from build123d import *

# Parameters (mm, degrees)
SKETCH2_R           = 15
SKETCH2_R_2         = 10
SKETCH5_R           = 5
CUT_EXTRUDE2_DEPTH  = 158.5
SKETCH6_R           = 30
CUT_EXTRUDE3_DEPTH  = 90.8
SKETCH9_R           = 10
BOSS_EXTRUDE2_DEPTH = 211.8
SKETCH10_R          = 4.5
BOSS_EXTRUDE3_DEPTH = 10


with BuildPart() as part:
    # Sweep2: sweep along a path in Sketch1
    with BuildLine(Plane(origin=(0, 0, 0), x_dir=(0, 0, -1), z_dir=(1, 0, 0))) as sweep2_path:
        Line((0, 0), (304.8, 0))
        ThreePointArc((304.8, 0), (361.368542495, 23.431457505), (384.8, 80))
        Line((384.8, 80), (384.8, 1748.2))
        ThreePointArc((384.8, 1748.2), (361.368542495, 1804.768542495), (304.8, 1828.2))
        Line((304.8, 1828.2), (0, 1828.2))
    # Sketch2 → Sweep2 (sweep)
    with BuildSketch(Plane.XY):
        with Locations((0, 1828.2)):
            Circle(SKETCH2_R)
        with Locations((0, 1828.2)):
            Circle(SKETCH2_R_2, mode=Mode.SUBTRACT)
    sweep(path=sweep2_path.line)

    # Sketch5 → Cut-Extrude2 (cut, symmetric)
    with BuildSketch(Plane(origin=(0, 0, 0), x_dir=(1, 0, 0), z_dir=(0, 1, 0))):
        with Locations(Location((0, 30, 0), (0, 0, 270))):
            Circle(SKETCH5_R)
        with Locations(Location((0, 230, 0), (0, 0, 270))):
            Circle(SKETCH5_R)
    extrude(amount=CUT_EXTRUDE2_DEPTH, both=True, mode=Mode.SUBTRACT)

    # Sketch6 → Cut-Extrude3 (cut)
    with BuildSketch(Plane.XY):
        with Locations((0, 1828.2)):
            Circle(SKETCH6_R)
    extrude(amount=-CUT_EXTRUDE3_DEPTH, mode=Mode.SUBTRACT)

    # Sketch9 → Boss-Extrude2 (add)
    with BuildSketch(Plane.XY.offset(-90.8)):
        with Locations((0, 1828.2)):
            Circle(SKETCH9_R)
    extrude(amount=-BOSS_EXTRUDE2_DEPTH)

    # Sketch10 → Boss-Extrude3 (add)
    with BuildSketch(Plane.XY.offset(-90.8)):
        with Locations((0, 1828.2)):
            Circle(SKETCH10_R)
    extrude(amount=BOSS_EXTRUDE3_DEPTH)


solid = part.part
Could you check a few things on this model? Use its own coordinates, in mm. Coordinates: 2 decimals unless noted, no trailing zeros. Order: outer loops, then holes, each group sorted by start corner. A loop starts at its lowest first (then second) coordinate and runs counter-clockwise, first axis right, second up.
Q1. Will these pins go through, and if not, where does the flat tip stop? pin 1 (12 mm diameter, centred on x = -12, z = -170, fed in from +Y); pin 2 (1.5 mm diameter, centred on x = -5.5, z = -298.5, fed in from +Y); pin 3 (8 mm diameter, centred on x = 0, z = -230, fed in from -Y).
Q2. Thinking about a two-plate mould opening in Y: for faces 1 (the flat face through (-10, -3, 0)), 2 (the cylindrical face through (-3.252, 925.777, -370.157)), which applies, released by +Y, released by -Y, zero draft, split by the parting line, or undercut?
Q3. Suppose I cut it at B-B on y = 174. Please give me the cut outline in (x, z), and give its area (3 significant figures).
Q4. Suppose I cut it at C-C on z = -345.5. Give the number of separate pieces and of enclosed holes in the cut face, and give its area (3 significant figures).
Q5. Please list where these lines run through material, in increasing order: L1, parallel to Y at x = 0, z = -129; L2, parallel to Y at x = -1, z = -148.5; L3, parallel to Z at x = 0, y = 1220.
Q6. Suppose I cut it at A-A on z = -129. Please give me the cut outline in (x, y).
Answer:
1. pin 1: stops at y = 1841.95
1. pin 2: stops at y = 1842.43
1. pin 3: stops at y = 1813.2
2. face 1: zero draft
2. face 2: undercut
3. outline: circle Ø30 at (0, -384.8); hole circle Ø20 at (0, -384.8)
3. area: 393 mm2
4. separate pieces: 2
4. enclosed holes: 2
4. area: 921 mm2
5. L1: y = -15 to -10, 10 to 15, 1813.2 to 1843.2
5. L2: y = -14.97 to -9.95, 9.95 to 14.97, 1813.23 to 1843.17
5. L3: z = -399.8 to -394.8, -374.8 to -369.8
6. outline: circle Ø30 at (0, 0); circle Ø30 at (0, 1828.2); hole circle Ø20 at (0, 0)
